```python
from build123d import *

# Parameters (mm, degrees)
SKETCH_1_W          = 2.5
SKETCH_1_H          = 6.25
SKETCH_1_W_2        = 6.25
SKETCH_1_H_2        = 2.5
EXTRUDE_1_DEPTH     = 15
SKETCH_2_R          = 17.5
EXTRUDE_2_DEPTH     = 120
SKETCH_3_W          = 7
SKETCH_3_H          = 20
CUT_EXTRUDE_1_DEPTH = 3


with BuildPart() as part:
    # 草图1 → 凸台-拉伸1 (new body)
    with BuildSketch(Plane.XY):
        with Locations((0, 4.375)):
            Rectangle(SKETCH_1_W, SKETCH_1_H)
        with Locations((-4.375, 0)):
            Rectangle(SKETCH_1_W_2, SKETCH_1_H_2)
        with Locations((4.375, 0)):
            Rectangle(SKETCH_1_W_2, SKETCH_1_H_2)
        with Locations((0, -4.375)):
            Rectangle(SKETCH_1_W, SKETCH_1_H)
        Rectangle(SKETCH_1_W, SKETCH_1_H_2)
    extrude(amount=-EXTRUDE_1_DEPTH)

    # 草图2 → 凸台-拉伸2 (add)
    with BuildSketch(Plane.XY):
        Circle(SKETCH_2_R)
    extrude(amount=EXTRUDE_2_DEPTH)

    # 草图3 → 切除-拉伸1 (cut)
    with BuildSketch(Plane(origin=(0, 17.5, 0), x_dir=(1, 0, 0), z_dir=(0, 1, 0))):
        with Locations((0, -110)):
            Rectangle(SKETCH_3_W, SKETCH_3_H)
    extrude(amount=-CUT_EXTRUDE_1_DEPTH, mode=Mode.SUBTRACT)


solid = part.part
```
Read the model definition and answer for the solid it produces. Units are mm, in the model's axes. A direction names the side the tool comes from. Coordinates: 2 decimals unless noted, no trailing zeros. Write each loop counter-clockwise with the first axis right and the second up, starting at its lowest first coordinate (ties: lowest second). Pieces come first, ordered by that corner, then holes. Notation, with made-up numbers: (41, 84) - (73, 84) arc R32 cw to (73, 119) - close; hole circle Ø10 at (-11.5, 41). An arc over 180 degrees is marked (long way). Answer as a JSON object with one key per item and string values. Group by question number.
1. Each of these flat-tipped pins is pushed along its axis until it touches: P1, Ø10, axis at x = 6.5, y = -12.5, coming from the -Z side; P2, Ø1.3, axis at y = 16, z = 109.5, coming from the +X side; P3, Ø10, axis at y = 7, z = 20, coming from the -X side. Where does it stop, or does it pass through?
2. A cutting plane is placed at B-B (y = 0). Determine the outline of the cut face in (x, z), plus the area to 4 significant figures.
3. A cutting plane is placed at C-C (z = 55.5). Determine the outline of the cut face in (x, y), plus the area to 3 significant figures.
4. A cutting plane is placed at D-D (x = -5.5). Determine the outline of the cut face in (y, z).
5. Consider L1, parallel to Z at x = 7, y = -3.5; L2, parallel to Y at x = 3.5, z = -2; L3, parallel to X at y = 4.5, z = 101. Determine where each line is inside the solid, lowest interval first. Write a range as [from, to].
6. Which of the six approach directions +Z, -Z, +X, -X, +Y, -Y give full straight-line access (tool end or side, diameter ignored) to faces 1 (the flat face through (0, 14.5, 110)), 2 (the flat face through (-1.25, 4, -7)), 3 (the flat face through (7.5, 0, -7)), 4 (the flat face through (4, 1.25, -7))?
7. A cutting plane is placed at A-A (x = 0). Determine the outline of the cut face in (y, z), plus the area to 4 significant figures.
8. The mould has two halves that part along X. Classify faces 5 (the flat face through (1.25, -4, -7)), 6 (the flat face through (-4, 1.25, -7)), 7 (the flat face through (3.5, 16, 110)): +X half, -X half, draft (parallel to the pull), parting line (faces both ways), or undercut.
Worked out:
{
 "1": {"P1": "stops at z = 0", "P2": "stops at x = 8.4", "P3": "stops at x = -17.39"},
 "2": {"outline": "(-17.5, 0) - (-7.5, 0) - (-7.5, -15) - (7.5, -15) - (7.5, 0) - (17.5, 0) - (17.5, 120) - (-17.5, 120) - close", "area": "4,425 mm²"},
 "3": {"outline": "circle Ø35 at (0, 0)", "area": "962 mm²"},
 "4": {"outline": "(-16.61, 0) - (-1.25, 0) - (-1.25, -15) - (1.25, -15) - (1.25, 0) - (16.61, 0) - (16.61, 120) - (-16.61, 120) - close"},
 "5": {"L1": "z = [0, 120]", "L2": "y = [-1.25, 1.25]", "L3": "x = [-16.91, 16.91]"},
 "6": {"face 1": "+Z, +Y", "face 2": "-Z, -X, +Y", "face 3": "-Z, +X, +Y, -Y", "face 4": "-Z, +X, +Y"},
 "7": {"outline": "(-17.5, 0) - (-7.5, 0) - (-7.5, -15) - (7.5, -15) - (7.5, 0) - (17.5, 0) - (17.5, 100) - (14.5, 100) - (14.5, 120) - (-17.5, 120) - close", "area": "4,365 mm²"},
 "8": {"face 5": "+X half", "face 6": "draft", "face 7": "undercut"}
}
